```python
from build123d import *

# Parameters (mm, degrees)
SKETCH1_R           = 19.05
BOSS_EXTRUDE1_DEPTH = 3.175


with BuildPart() as part:
    # Sketch1 → Boss-Extrude1 (new body)
    with BuildSketch(Plane.XY):
        with BuildLine():
            Line((-19.05, -92.029005754), (-19.05, -88.774236431))
            Line((-19.05, -88.774236431), (-15.875, -88.774236431))
            Line((-15.875, -88.774236431), (-15.875, -92.629502725))
            ThreePointArc((-15.875, -92.629502725), (0, -93.98), (15.875, -92.629502725))
            Line((15.875, -92.629502725), (15.875, -88.774236431))
            Line((15.875, -88.774236431), (19.05, -88.774236431))
            Line((19.05, -88.774236431), (19.05, -92.029005754))
            ThreePointArc((19.05, -92.029005754), (20.640594227, -91.685365626), (22.225, -91.314236431))
            ThreePointArc((22.225, -91.314236431), (67.594559133, -65.29330728), (92.029005754, -19.05))
            Line((92.029005754, -19.05), (88.774236431, -19.05))
            Line((88.774236431, -19.05), (88.774236431, -15.875))
            Line((88.774236431, -15.875), (92.629502725, -15.875))
            ThreePointArc((92.629502725, -15.875), (93.98, 0), (92.629502725, 15.875))
            Line((92.629502725, 15.875), (88.774236431, 15.875))
            Line((88.774236431, 15.875), (88.774236431, 19.05))
            Line((88.774236431, 19.05), (92.029005754, 19.05))
            ThreePointArc((92.029005754, 19.05), (66.453895296, 66.453895296), (19.05, 92.029005754))
            Line((19.05, 92.029005754), (19.05, 88.774236431))
            Line((19.05, 88.774236431), (15.875, 88.774236431))
            Line((15.875, 88.774236431), (15.875, 92.629502725))
            ThreePointArc((15.875, 92.629502725), (0, 93.98), (-15.875, 92.629502725))
            Line((-15.875, 92.629502725), (-15.875, 88.774236431))
            Line((-15.875, 88.774236431), (-19.05, 88.774236431))
            Line((-19.05, 88.774236431), (-19.05, 92.029005754))
            ThreePointArc((-19.05, 92.029005754), (-20.640594227, 91.685365626), (-22.225, 91.314236431))
            ThreePointArc((-22.225, 91.314236431), (-66.453895296, 66.453895296), (-91.314236431, 22.225))
            ThreePointArc((-91.314236431, 22.225), (-91.685365626, 20.640594227), (-92.029005754, 19.05))
            Line((-92.029005754, 19.05), (-88.774236431, 19.05))
            Line((-88.774236431, 19.05), (-88.774236431, 15.875))
            Line((-88.774236431, 15.875), (-92.629502725, 15.875))
            ThreePointArc((-92.629502725, 15.875), (-93.98, 0), (-92.629502725, -15.875))
            Line((-92.629502725, -15.875), (-88.774236431, -15.875))
            Line((-88.774236431, -15.875), (-88.774236431, -19.05))
            Line((-88.774236431, -19.05), (-92.029005754, -19.05))
            ThreePointArc((-92.029005754, -19.05), (-66.453895296, -66.453895296), (-19.05, -92.029005754))
        make_face()
        Circle(SKETCH1_R, mode=Mode.SUBTRACT)
    extrude(amount=BOSS_EXTRUDE1_DEPTH)


solid = part.part
```
Could you check a few things on this model? Use its own coordinates, in mm. Give positions to 0.01 mm unless a question says otherwise; leave off trailing zeros. Order: outer loops, then holes, each group sorted by start corner. A loop starts at its lowest first (then second) coordinate and runs counter-clockwise, first axis right, second up.
Q1. Suppose I cut it at B-B, the plane y = -13.5. Write out the boundary of the cut face in (x, z) (3 decimals), and give its area (3 significant figures).
Q2. If I drill on line 1 along Y through (x, z) = (-22, 2.6); line 2 along Y through (x, z) = (-3, 1.3); line 3 along X through (y, z) = (76.5, 2.4), over which ranges is the centre line in solid material (lowest first)?
Q3. Suppose I cut it at C-C, the plane x = 42.5. Write out the boundary of the cut face in (y, z) (3 decimals), and give its area (3 significant figures).
Q4. Suppose I cut it at A-A, the plane x = 0. Write out the boundary of the cut face in (y, z) (3 decimals).
Q5. Suppose I cut it at D-D, the plane x = -60. Write out the boundary of the cut face in (y, z) (3 decimals), and give its area (3 significant figures).
Q6. I'm going to push flat-ended pins straight in: P1, Ø1.6, axis at x = 17, z = 2, coming from the -Y side; P2, Ø1.5, axis at y = -5.5, z = 2, coming from the -X side. Where does each tip first touch, or does it pass through?
Q7. We'd pull the mould along Y, two halves only. Please class faces 1 (the cylindrical face through (-66.992, -65.911, 1.565)), 2 (the cylindrical face through (-15.12, -11.59, 1.57)), 3 (the flat face through (-1, -20, 0)): +Y half, -Y half, draft (parallel to the pull), parting line (faces both ways), or undercut.
Solution:
1. outline: (-93.005, 0) - (-13.441, 0) - (-13.441, 3.175) - (-93.005, 3.175) - close; (13.441, 0) - (93.005, 0) - (93.005, 3.175) - (13.441, 3.175) - close
1. area: 505 mm2
2. line 1: y = -91.37 to 91.37
2. line 2: y = -93.93 to -18.81, 18.81 to 93.93
2. line 3: x = -54.59 to 54.59
3. outline: (-83.821, 0) - (83.821, 0) - (83.821, 3.175) - (-83.821, 3.175) - close
3. area: 532 mm2
4. outline: (-93.98, 0) - (-19.05, 0) - (-19.05, 3.175) - (-93.98, 3.175) - close; (19.05, 0) - (93.98, 0) - (93.98, 3.175) - (19.05, 3.175) - close
5. outline: (-72.334, 0) - (72.334, 0) - (72.334, 3.175) - (-72.334, 3.175) - close
5. area: 459 mm2
6. P1: stops at y = -88.77
6. P2: stops at x = -93.86
7. face 1: -Y half
7. face 2: undercut
7. face 3: draft
